```python
from build123d import *

# Parameters (mm, degrees)
SKETCH1_W           = 83
SKETCH1_H           = 62
BOSS_EXTRUDE1_DEPTH = 5
SKETCH2_W           = 15
SKETCH2_H           = 10
CUT_EXTRUDE1_DEPTH  = 10
CUT_EXTRUDE2_DEPTH  = 5


with BuildPart() as part:
    # Sketch1 → Boss-Extrude1 (new body)
    with BuildSketch(Plane.XY):
        Rectangle(SKETCH1_W, SKETCH1_H)
    extrude(amount=BOSS_EXTRUDE1_DEPTH)

    # Sketch2 → Cut-Extrude1 (cut)
    with BuildSketch(Plane.XY.offset(5)):
        with Locations((34, -26)):
            Rectangle(SKETCH2_W, SKETCH2_H)
    extrude(amount=-CUT_EXTRUDE1_DEPTH, mode=Mode.SUBTRACT)

    # Sketch3 → Cut-Extrude2 (cut)
    with BuildSketch(Plane.XY.offset(5)):
        Polygon((-27.1, 22.6), (-27.1, 12.6), (-31.5, 12.6), (-31.5, 22.6), (-33, 22.6), (-33, 26), (-31.5, 26), (-31.5, 31), (-27.1, 31), (-27.1, 26), (-25.6, 26), (-25.6, 22.6), align=None)
        Polygon((31.5, 12.6), (31.5, 22.6), (33, 22.6), (33, 26), (31.5, 26), (31.5, 31), (27.1, 31), (27.1, 26), (25.6, 26), (25.6, 22.6), (27.1, 22.6), (27.1, 12.6), align=None)
        Polygon((-31.5, -12.6), (-31.5, -22.6), (-33, -22.6), (-33, -26), (-31.5, -26), (-31.5, -31), (-27.1, -31), (-27.1, -26), (-25.6, -26), (-25.6, -22.6), (-27.1, -22.6), (-27.1, -12.6), align=None)
    extrude(amount=-CUT_EXTRUDE2_DEPTH, mode=Mode.SUBTRACT)


solid = part.part
```
Here's how the part is built. I have some questions about the finished solid (model axes, mm). A direction names the side the tool comes from. Round coordinates to 2 decimals unless told otherwise and drop trailing zeros. Loops run counter-clockwise (first coordinate to the right, second up) from the corner with the lowest first, then second, coordinate; pieces in that order, holes last.
1. Thinking about a two-plate mould opening in Y: for faces 1 (the face through (-29, 12.6, 3)), 2 (the face through (-27.1, -29, 3)), 3 (the face through (-25.6, -24, 3)), 4 (the face through (-37, -31, 2)), which applies, released by +Y, released by -Y, zero draft, split by the parting line, or undercut?
Answers:
face 1: released by +Y
face 2: zero draft
face 3: undercut
face 4: released by -Y
2. For faces 5 (the face through (0, 31, 2)), 6 (the face through (-31.5, -28, 3)), 7 (the face through (25.6, 24, 3)), 8 (the face through (41.5, 5, 2)), 9 (the face through (-27.1, 29, 3)), which set-ups out of +Z, -Z, +X, -X, +Y, -Y let a thin tool reach every point of the face, with its end or its side?
Answers:
face 5: +Z, -Z, +X, -X, +Y
face 6: +Z, -Z, -Y
face 7: +Z, -Z
face 8: +Z, -Z, +X, +Y, -Y
face 9: +Z, -Z, +Y
3. Suppose I cut it at A-A, the plane y = -14. Please give me the cut outline in (x, z).
Answers:
outline: (-41.5, 0) - (-31.5, 0) - (-31.5, 5) - (-41.5, 5) - close; (-27.1, 0) - (41.5, 0) - (41.5, 5) - (-27.1, 5) - close
4. Will this pin go through, and if not, where does the flat tip stop? pin 1 (1.3 mm diameter, centred on x = 29, z = 2.5, fed in from +Y).
Answers:
pin 1: stops at y = 12.6
5. Suppose I cut it at B-B, the plane y = 19.5. Please give me the cut outline in (x, z), and give its area (3 significant figures).
Answers:
outline: (-41.5, 0) - (-31.5, 0) - (-31.5, 5) - (-41.5, 5) - close; (-27.1, 0) - (27.1, 0) - (27.1, 5) - (-27.1, 5) - close; (31.5, 0) - (41.5, 0) - (41.5, 5) - (31.5, 5) - close
area: 371 mm2
6. Suppose I cut it at C-C, the plane x = 28.5. Please give me the cut outline in (y, z), and give its area (3 significant figures).
Answers:
outline: (-21, 0) - (12.6, 0) - (12.6, 5) - (-21, 5) - close
area: 168 mm2
7. If I drill on probe 1 along X at (y, z) = (20, 2.9); probe 2 along Y at (x, z) = (37, 0.7); probe 3 along X at (y, z) = (-16, 1.1), over which ranges is the centre line in solid material (lowest first)?
Answers:
probe 1: x = -41.5 to -31.5, -27.1 to 27.1, 31.5 to 41.5
probe 2: y = -21 to 31
probe 3: x = -41.5 to -31.5, -27.1 to 41.5
